Design review of the part shown in the three views and the two pictorial views. Dimensions are in mm from the part's minimum x, y and z. A direction names the side the tool comes from. Round coordinates to 2 decimals unless told otherwise and drop trailing zeros. Loops run counter-clockwise (first coordinate to the right, second up) from the corner with the lowest first, then second, coordinate; pieces in that order, holes last. Notation, with made-up numbers: M -1,31 L 6,31 A23 cw 6,45 Z; hole C 6.5,19 d6. An arc over 180 degrees is marked long. One line per question, with ' | ' between items.
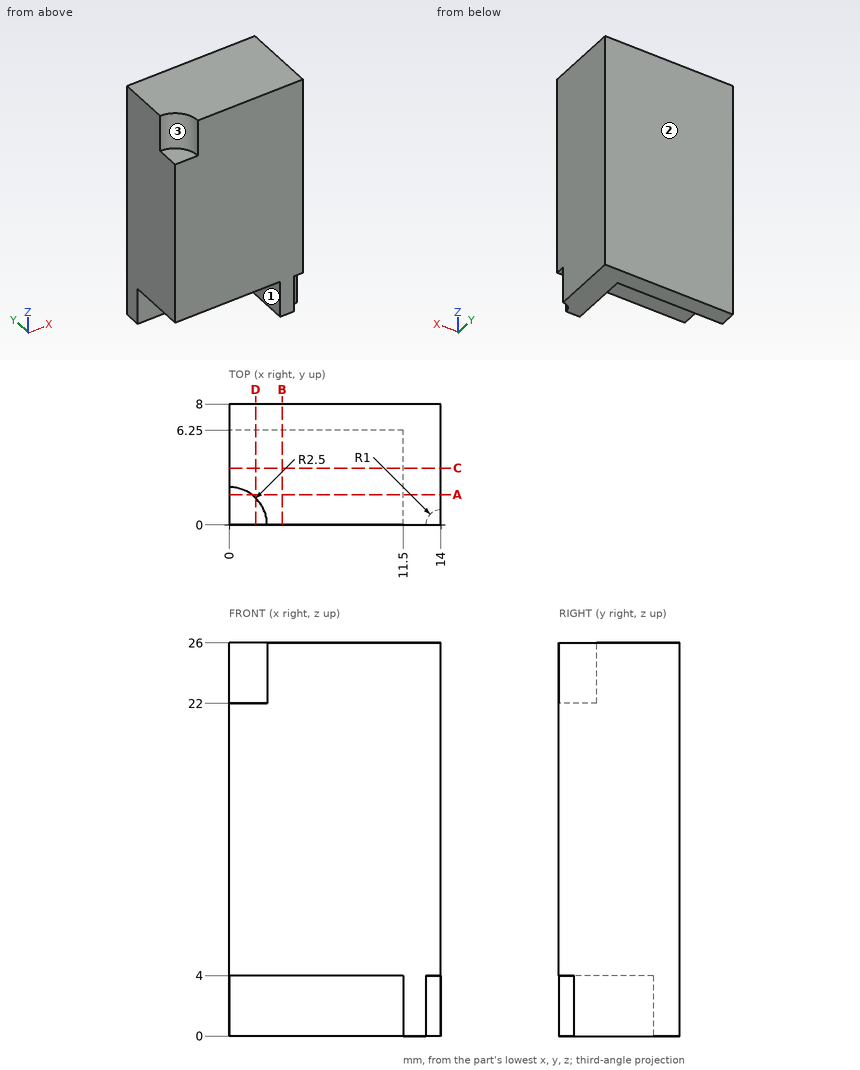
1) Add section C-C on y = 3.75. State the section outline as (x, z) points.
Output values:
outline: M 0,4 L 11.5,4 L 11.5,0 L 14,0 L 14,26 L 0,26 Z
2) For line 1 (Z direction, x = 4.25, y = 2.5); line 2 (Y direction, x = 2, z = 2.75); line 3 (Z direction, x = 1, y = 1), list the stretches that pass through material, from the lowest coordinate up.
Output values:
line 1: z = 4 to 26 | line 2: y = 6.25 to 8 | line 3: z = 4 to 22
3) Insertion check: P1, Ø2, axis at x = 3.5, z = 1.5, coming from the -Y side. The pin has a flat end and moves straight along its axis. Give the tip position at first contact, or say it passes through.
Output values:
P1: stops at y = 6.25
4) Add section A-A on y = 2. State the section outline as (x, z) points.
Output values:
outline: M 0,4 L 11.5,4 L 11.5,0 L 14,0 L 14,26 L 1.5,26 L 1.5,22 L 0,22 Z
5) Machinability: for the marked faces 1, 2 and 3, which of the approach directions +Z, -Z, +X, -X, +Y, -Y give a long, thin tool a straight path to every point of the face, cutting with its end or side? Answer none if there is none.
Output values:
face 1: -Z, -X, -Y | face 2: +Z, -Z, +X, -X, +Y | face 3: +Z, -X, -Y
6) Add section D-D on x = 1.75. State the section outline as (y, z) points, then the cut area to 3 significant figures.
Output values:
outline: M 0,4 L 6.25,4 L 6.25,0 L 8,0 L 8,26 L 1.79,26 L 1.79,22 L 0,22 Z | area: 176 mm²
7) Add section B-B on x = 3.5. State the section outline as (y, z) points, then the cut area to 3 significant figures.
Output values:
outline: M 0,4 L 6.25,4 L 6.25,0 L 8,0 L 8,26 L 0,26 Z | area: 183 mm²
